The model under review builds one solid part; all positions refer to its coordinate system, in mm. Face numbers are marked on the shaded views. A direction names the side the tool comes from. Coordinates: 2 decimals unless noted, no trailing zeros. Loops run counter-clockwise (first coordinate to the right, second up) from the corner with the lowest first, then second, coordinate; pieces in that order, holes last. Notation, with made-up numbers: (83.25, 1) - (116.25, 1) arc R22 cw to (116.25, 37) - close; hole circle Ø4 at (37, -8.75). An arc over 180 degrees is marked (long way). Use a Markdown table: item, result. Add a question column.
1) Add section B-B, the plane x = 1. Give the boundary of the cut face in (y, z), and give its area (3 significant figures).
2) To check wall thickness, follow L1, parallel to X at y = 0, z = 36.75; L2, parallel to Y at x = -2, z = 33.5; L3, parallel to X at y = 0, z = 33.75. State the ranges of each line that lie inside material, in increasing order. Write a range as [from, to].
3) Add section A-A, the plane y = 0. Give the boundary of the cut face in (x, z), and give its area (3 significant figures).
4) Clearance check with flat-ended pins moving along their axes: pin 1 (4 mm diameter, centred on x = -2.5, z = 30, fed in from -Y); pin 2 (1.5 mm diameter, centred on y = 0, z = 33, fed in from +X); pin 3 (2 mm diameter, centred on x = -1.5, y = 2.5, fed in from +Z); pin 4 (1.5 mm diameter, centred on x = 1.5, z = 37, fed in from -Y). State where each tip first meets the part, or that it passes through.
5) For the marked faces 4, 5 and 6, list the 3-axis set-ups (+Z, -Z, +X, -X, +Y, -Y) from which the entire face can be reached by the end or side of a thin tool; tool diameter is ignored.
6) The part is to be moulded in two halves that separate along Z. For the marked faces 1, 2 and 3, say which applies: pulls with the +Z half, pulls with the -Z half, needs draft (parallel to the pull), parting line crosses it, or undercut.
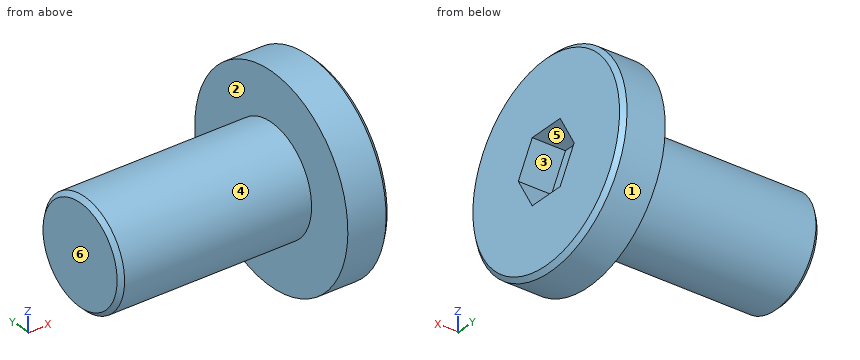
```python
from build123d import *

# Parameters (mm, degrees)
F0_W     = 9
F0_H     = 2.5
F2_SIZE  = 0.2
F4_DEPTH = 1.56


with BuildPart() as f1:
    # F0 (on Front) → F1 (revolve)
    with BuildSketch(Plane.XZ):
        with Locations((-0.4593508661, 34.7560998052)):
            Rectangle(F0_W, F0_H)
        Polygon((4.0406491339, 38.2560998052), (4.0406491339, 36.0060998052), (4.0406491339, 33.5060998052), (6.0406491339, 33.5060998052), (6.0406491339, 38.2560998052), align=None)
    revolve(axis=Axis((-0.4593508661, 0, 33.5060998052), (-1, 0, 0)))

    # F2
    f2_edges = [f1.edges().sort_by_distance(p)[0] for p in [
        (-4.959351, 0, 31.0061),
        (6.040649, 0, 28.7561),
    ]]
    chamfer(f2_edges, length=F2_SIZE)

    # F3 (on face) → F4 (cut)
    with BuildSketch(Plane.YZ.offset(6.0406491339)):
        Polygon((0.8660254038, 35.0060998052), (-0.8660254038, 35.0060998052), (-1.7320508076, 33.5060998052), (-0.8660254038, 32.0060998052), (0.8660254038, 32.0060998052), (1.7320508076, 33.5060998052), align=None)
    extrude(amount=-F4_DEPTH, mode=Mode.SUBTRACT)


solid = f1.part
```
From the geometry:
| question | item | result |
|---|---|---|
| 1 | outline | circle Ø5 at (0, 33.51) |
| 1 | area | 19.6 mm^2 |
| 2 | L1 | x = [4.04, 6.04] |
| 2 | L2 | y = [-2.5, 2.5] |
| 2 | L3 | x = [-4.96, 4.48] |
| 3 | outline | (-4.96, 31.21) - (-4.76, 31.01) - (4.04, 31.01) - (4.04, 28.76) - (5.84, 28.76) - (6.04, 28.96) - (6.04, 32.01) - (4.48, 32.01) - (4.48, 35.01) - (6.04, 35.01) - (6.04, 38.06) - (5.84, 38.26) - (4.04, 38.26) - (4.04, 36.01) - (-4.76, 36.01) - (-4.96, 35.81) - close |
| 3 | area | 59.2 mm^2 |
| 4 | pin 1 | stops at y = -2 |
| 4 | pin 2 | stops at x = 4.48 |
| 4 | pin 3 | stops at z = 35.51 |
| 4 | pin 4 | passes through |
| 5 | face 4 | -X |
| 5 | face 5 | +X |
| 5 | face 6 | +Z, -Z, -X, +Y, -Y |
| 6 | face 1 | parting line crosses it |
| 6 | face 2 | needs draft |
| 6 | face 3 | undercut |
